Build history of the part. All positions in model axes, mm. Round coordinates to 2 decimals unless told otherwise and drop trailing zeros. Write each loop counter-clockwise with the first axis right and the second up, starting at its lowest first coordinate (ties: lowest second). Pieces come first, ordered by that corner, then holes.
1) Saw through at B-B (z = 35). Write the cut outline in (x, y), plus the area to 3 significant figures.
2) Wall check: probe 1 along X at (y, z) = (2, 0); probe 2 along X at (y, z) = (1.8, 35). Give the ranges that are in metal, low to high.
3) Flat gauge pins, fed straight in: pin 1 (4.5 mm diameter, centred on x = 49, z = -10, fed in from -Y); pin 2 (4 mm diameter, centred on x = 25.5, z = 0, fed in from -Y). Where does each tip first touch, or does it go through?
4) Saw through at D-D (x = 0). Write the cut outline in (y, z).
5) Saw through at C-C (y = 0.85). State how many separate pieces and enclosed holes the cut face has, plus the area to 3 significant figures.
6) Saw through at A-A (x = -25.5). Write the cut outline in (y, z), plus the area to 3 significant figures.
from build123d import *

# Parameters (mm, degrees)
SKETCH_1_W          = 110
SKETCH_1_H          = 110
EXTRUDE_1_DEPTH     = 4
SKETCH_2_R          = 2.6
CUT_EXTRUDE_1_DEPTH = 78.884529914
SKETCH_3_R          = 1.5
CUT_EXTRUDE_2_DEPTH = 78.884529914
SKETCH_4_R          = 2.6
CUT_EXTRUDE_3_DEPTH = 78.884529914


with BuildPart() as part:
    # 草图1 → 凸台-拉伸1 (new body)
    with BuildSketch(Plane(origin=(0, 0, 0), x_dir=(1, 0, 0), z_dir=(0, 1, 0))):
        Rectangle(SKETCH_1_W, SKETCH_1_H)
    extrude(amount=EXTRUDE_1_DEPTH)

    # 草图2 → 切除-拉伸1 (cut, through all)
    with BuildSketch(Plane(origin=(0, 0, 0), x_dir=(1, 0, 0), z_dir=(0, 1, 0))):
        with Locations(Location((0, 35, 0), (0, 0, 270))):
            Circle(SKETCH_2_R)
        with Locations(Location((35, 0, 0), (0, 0, 270))):
            Circle(SKETCH_2_R)
        with Locations(Location((0, -35, 0), (0, 0, 270))):
            Circle(SKETCH_2_R)
        with Locations(Location((-35, 0, 0), (0, 0, 270))):
            Circle(SKETCH_2_R)
    extrude(amount=CUT_EXTRUDE_1_DEPTH, mode=Mode.SUBTRACT)

    # 草图3 → 切除-拉伸2 (cut, through all)
    with BuildSketch(Plane(origin=(0, 4, 0), x_dir=(1, 0, 0), z_dir=(0, 1, 0))):
        with Locations(Location((0, 25.5, 0), (0, 0, 270))):
            Circle(SKETCH_3_R)
        with Locations(Location((25.5, 0, 0), (0, 0, 270))):
            Circle(SKETCH_3_R)
        with Locations(Location((0, -25.5, 0), (0, 0, 270))):
            Circle(SKETCH_3_R)
        with Locations(Location((-25.5, 0, 0), (0, 0, 270))):
            Circle(SKETCH_3_R)
    extrude(amount=-CUT_EXTRUDE_2_DEPTH, mode=Mode.SUBTRACT)

    # 草图4 → 切除-拉伸3 (cut, through all)
    with BuildSketch(Plane(origin=(0, 4, 0), x_dir=(1, 0, 0), z_dir=(0, 1, 0))):
        with Locations(Location((-10, 49, 0), (0, 0, 270))):
            Circle(SKETCH_4_R)
        with Locations(Location((10, 49, 0), (0, 0, 270))):
            Circle(SKETCH_4_R)
        with Locations(Location((49, 10, 0), (0, 0, 270))):
            Circle(SKETCH_4_R)
        with Locations(Location((49, -10, 0), (0, 0, 270))):
            Circle(SKETCH_4_R)
        with Locations(Location((10, -49, 0), (0, 0, 270))):
            Circle(SKETCH_4_R)
        with Locations(Location((-10, -49, 0), (0, 0, 270))):
            Circle(SKETCH_4_R)
        with Locations(Location((-49, -10, 0), (0, 0, 270))):
            Circle(SKETCH_4_R)
        with Locations(Location((-49, 10, 0), (0, 0, 270))):
            Circle(SKETCH_4_R)
    extrude(amount=-CUT_EXTRUDE_3_DEPTH, mode=Mode.SUBTRACT)


solid = part.part
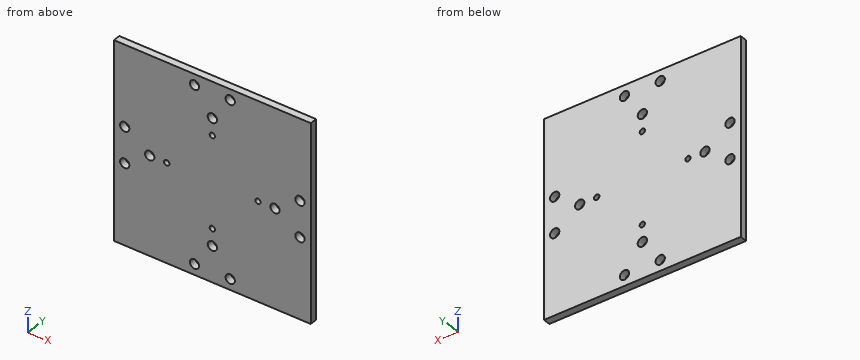
Evaluation:
1. outline: (-55, 0) - (-2.6, 0) - (-2.6, 4) - (-55, 4) - close; (2.6, 0) - (55, 0) - (55, 4) - (2.6, 4) - close
1. area: 419 mm2
2. probe 1: x = -55 to -37.6, -32.4 to -27, -24 to 24, 27 to 32.4, 37.6 to 55
2. probe 2: x = -55 to -2.6, 2.6 to 55
3. pin 1: passes through
3. pin 2: stops at y = 0
4. outline: (0, -55) - (4, -55) - (4, -37.6) - (0, -37.6) - close; (0, -32.4) - (4, -32.4) - (4, -27) - (0, -27) - close; (0, -24) - (4, -24) - (4, 24) - (0, 24) - close; (0, 27) - (4, 27) - (4, 32.4) - (0, 32.4) - close; (0, 37.6) - (4, 37.6) - (4, 55) - (0, 55) - close
5. separate pieces: 1
5. enclosed holes: 16
5. area: 11,800 mm2
6. outline: (0, -55) - (4, -55) - (4, -1.5) - (0, -1.5) - close; (0, 1.5) - (4, 1.5) - (4, 55) - (0, 55) - close
6. area: 428 mm2
